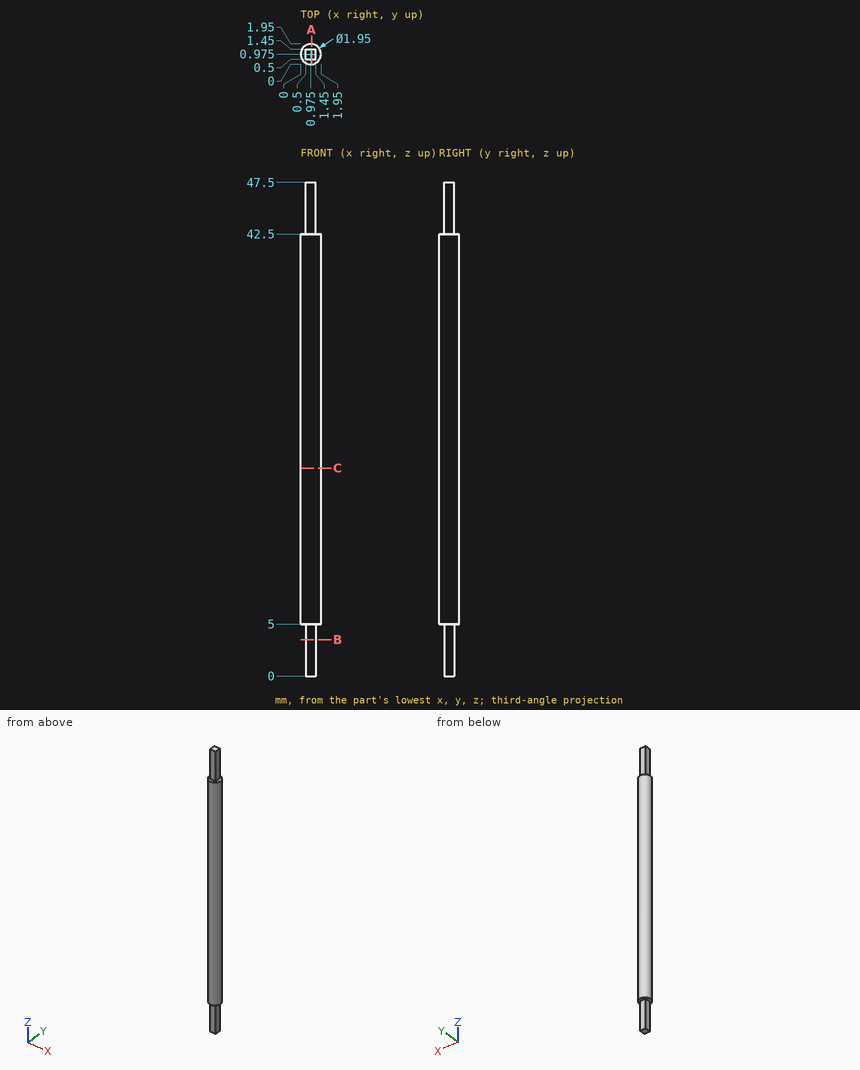
The figure shows three views and two pictorial views of one solid part (mm, origin at its lowest corner). Answer the questions. Give positions to 0.01 mm unless a question says otherwise; leave off trailing zeros. Write each loop counter-clockwise with the first axis right and the second up, starting at its lowest first coordinate (ties: lowest second). Pieces come first, ordered by that corner, then holes. Notation, with made-up numbers: (26, 83.5) -> (33, 83.5) arc R31 ccw to (33, 108.5) -> close; hole circle Ø10 at (26.5, -26). An arc over 180 degrees is marked (long way). Write each question's results on one line, items separated by ' | '.
1. Each of these flat-tipped pins is pushed along its axis until it touches: pin 1 Ø0.5 at (x, z) = (1, 3) entering from +Y; pin 2 Ø0.5 at (y, z) = (1, 1.5) entering from -X; pin 3 Ø1 at (y, z) = (1, 45.5) entering from +X. Where does it stop, or does it pass through?
Data:
pin 1: y = 1.45 | pin 2: x = 0.5 | pin 3: x = 1.45
2. Find section B-B on z = 3.5. Determine the outline of the cut face in (x, y).
Data:
outline: (0.5, 0.5) -> (1.45, 0.5) -> (1.45, 1.45) -> (0.5, 1.45) -> close
3. Find section A-A on x = 1.05. Determine the outline of the cut face in (y, z), and give its area (3 significant figures).
Data:
outline: (0, 5) -> (0.5, 5) -> (0.5, 0) -> (1.45, 0) -> (1.45, 5) -> (1.95, 5) -> (1.95, 42.5) -> (1.45, 42.5) -> (1.45, 47.5) -> (0.5, 47.5) -> (0.5, 42.5) -> (0, 42.5) -> close | area: 82.4 mm^2
4. Find section C-C on z = 20. Determine the outline of the cut face in (x, y) (3 decimals).
Data:
outline: circle Ø1.95 at (0.975, 0.975)
5. Straight lines are drawn through the part: L1, parallel to Z at x = 0.65, y = 0.25; L2, parallel to X at y = 0.85, z = 43.5; L3, parallel to X at y = 0.85, z = 12. For each, find the intervals that lie inside material, in ascending order.
Data:
L1: 5 to 42.5 | L2: 0.5 to 1.45 | L3: 0.01 to 1.94
